Source: three-view drawing plus pictorial views. Frame: mm from the lowest corner of the part. Round coordinates to 2 decimals unless told otherwise and drop trailing zeros. Loops run counter-clockwise (first coordinate to the right, second up) from the corner with the lowest first, then second, coordinate; pieces in that order, holes last. Notation, with made-up numbers: (54, 41) -> (59, 41) arc R13 cw to (59, 64) -> close; hole circle Ø10 at (36.5, 53). An arc over 180 degrees is marked (long way). Answer in a Markdown table with one row per item.
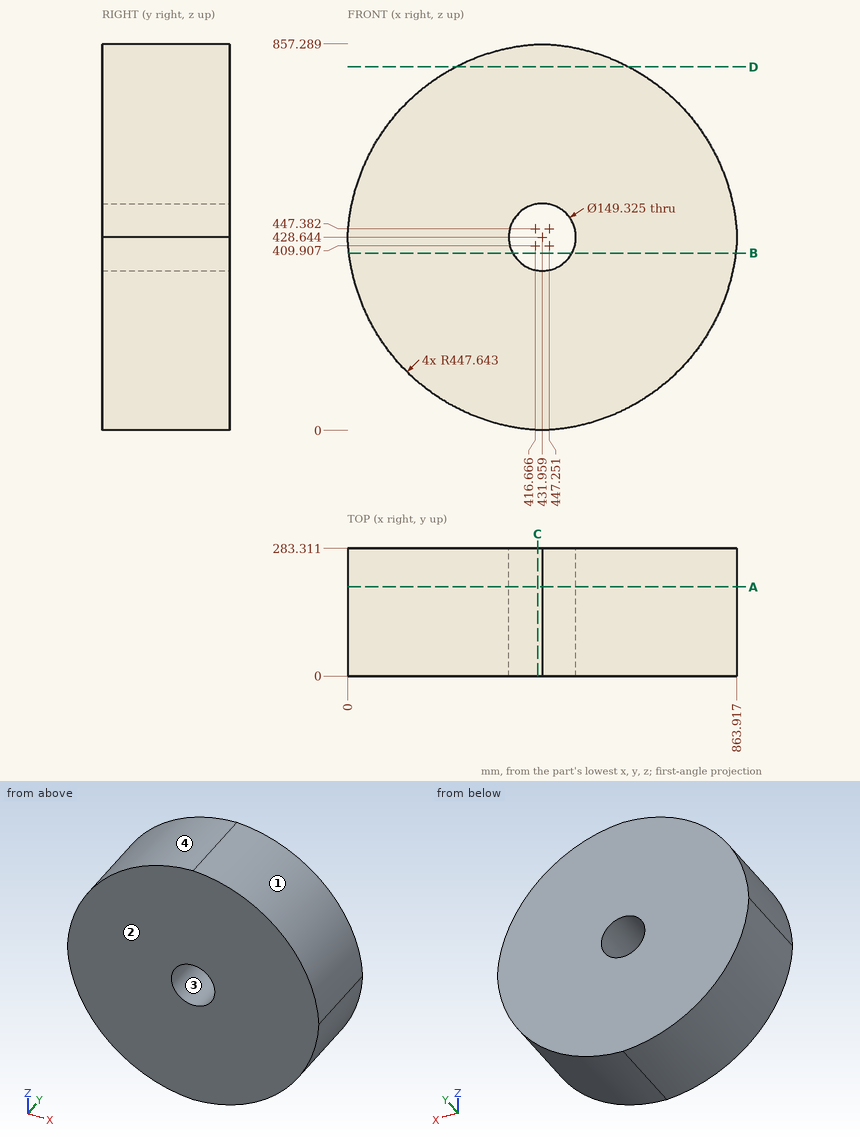
Item 1: Draft query along X for the marked faces 1, 2, 3 and 4. Return one class per face: pulls with the +X half, pulls with the -X half, needs draft (parallel to the pull), parting line crosses it, or undercut.
Answer:
| item | result |
|---|---|
| face 1 | pulls with the +X half |
| face 2 | needs draft |
| face 3 | undercut |
| face 4 | pulls with the -X half |
Item 2: Pin query (flat end, axial travel): pin 1 Ø1 at (x, y) = (262, 165) entering from +Z; pin 2 Ø8 at (y, z) = (146, 249.5) entering from +X (1 decimal); pin 3 Ø10 at (y, z) = (117, 655) entering from +X (1 decimal). Return the tip coordinate at first contact, or that it passes through.
Answer:
| item | result |
|---|---|
| pin 1 | stops at z = 817.65 |
| pin 2 | stops at x = 820.1 |
| pin 3 | stops at x = 794.5 |
Item 3: Cut plane B-B (z = 393). Output: boundary loops of the cut face in (x, y) (1 decimal), then the cut area to 3 significant figures.
Answer:
| item | result |
|---|---|
| outline | (2.9, 0) -> (366.4, 0) -> (366.4, 283.3) -> (2.9, 283.3) -> close; (497.6, 0) -> (861, 0) -> (861, 283.3) -> (497.6, 283.3) -> close |
| area | 206,000 mm² |
Item 4: Cut plane A-A (y = 198). Output: boundary loops of the cut face in (x, z) (1 decimal), then the cut area to 3 significant figures.
Answer:
| item | result |
|---|---|
| outline | (0, 428.6) arc R447.6 ccw to (432, 0) arc R447.6 ccw to (863.9, 428.6) arc R447.6 ccw to (432, 857.3) arc R447.6 ccw to start; hole circle Ø149.3 at (432, 428.6) |
| area | 552,000 mm² |
Item 5: Cut plane D-D (z = 806.5). Output: boundary loops of the cut face in (x, y).
Answer:
| item | result |
|---|---|
| outline | (239.65, 0) -> (624.27, 0) -> (624.27, 283.31) -> (239.65, 283.31) -> close |
Item 6: Cut plane C-C (x = 421.5). Output: boundary loops of the cut face in (y, z), then the cut area to 3 significant figures.
Answer:
| item | result |
|---|---|
| outline | (0, 0.48) -> (283.31, 0.48) -> (283.31, 354.72) -> (0, 354.72) -> close; (0, 502.57) -> (283.31, 502.57) -> (283.31, 856.81) -> (0, 856.81) -> close |
| area | 201,000 mm² |
Item 7: Line query: probe 1 along X at (y, z) = (13.5, 429) (1 decimal); probe 2 along Z at (x, y) = (445, 260) (1 decimal); probe 3 along X at (y, z) = (131, 749) (1 decimal). Output: solid intervals per line, ascending. Write a range as [from, to].
Answer:
| item | result |
|---|---|
| probe 1 | x = [0, 357.3], [506.6, 863.9] |
| probe 2 | z = [0.6, 355.1], [502.2, 856.7] |
| probe 3 | x = [155, 708.9] |
